Could you check a few things on this model? Use its own coordinates, in mm. A direction names the side the tool comes from. Give positions to 0.01 mm unless a question says otherwise; leave off trailing zeros. Loops run counter-clockwise (first coordinate to the right, second up) from the corner with the lowest first, then second, coordinate; pieces in that order, holes last. Notation, with made-up numbers: (69.5, 2.5) -> (92.5, 2.5) arc R28 cw to (92.5, 24.5) -> close; hole circle Ø2 at (-25.5, -22.75). An arc over 180 degrees is marked (long way). Write item = value, one per line. Start each with the question number.
1) I need wall thicknesses on probe 1 along Z at (x, y) = (19.5, -1.3) (3 decimals); probe 2 along X at (y, z) = (-1, -124) (3 decimals); probe 3 along X at (y, z) = (-2.6, -128) (3 decimals). Which ranges of each line are inside material? Lowest first, please. Write a range as from..to.
2) I want a section at B-B (x = -106). List the corners of the cut face in (y, z) for me (3 decimals).
3) On a 3-axis mill with a long thin cutter (end or side, diameter ignored), from which of +Z, -Z, +X, -X, +Y, -Y can I reach the whole of each face in a straight line? I mean faces 1 (the face through (77.401, -1.565, -75.264)), 2 (the face through (265.049, -1.565, -262.944)). Say none if no direction works.
4) I'm going to push flat-ended pins straight in: pin 1 Ø1.6 at (x, y) = (-361, -1) entering from +Z (3 decimals); pin 2 Ø6 at (x, z) = (-29, -121.5) entering from -Y (3 decimals). Where does each tip first touch, or does it pass through?
5) If we mould it in two halves opening along Z, with no side actions, what happens to faces 3 (the face through (-75.264, -1.565, -77.401)), 4 (the face through (262.944, -1.565, 265.049)), 5 (the face through (79, -3.175, -89))? For each: +Z half, -Z half, draft (parallel to the pull), parting line (faces both ways), or undercut.
6) I want a section at C-C (z = 65). List the corners of the cut face in (x, y) for me (3 decimals), and give its area (3 significant figures).
7) I want a section at D-D (x = -221.5). List the corners of the cut face in (y, z) for me (3 decimals), and give its area (3 significant figures).
8) I want a section at A-A (y = -2.3). List the corners of the cut face in (x, z) for me (3 decimals).
from build123d import *

# Parameters (mm, degrees)
SKETCH2_W           = 755.65
SKETCH2_H           = 755.65
BASE_FLANGE1_DEPTH  = 3.175
CUT_EXTRUDE1_DEPTH  = 535.334672162
CUT_EXTRUDE2_DEPTH  = 535.334672162
BREAK_CORNER1_START = -3.175
BREAK_CORNER1_DEPTH = 3.175


# Read off the part's stored shape, not the designer's step: Break-Corner1
# Sheet-metal steps are written as plain solids
with BuildPart() as part:
    # Sketch2 → Base-Flange1 (new body)
    with BuildSketch(Plane(origin=(0, 0, 0), x_dir=(1, 0, 0), z_dir=(0, 1, 0))):
        Rectangle(SKETCH2_W, SKETCH2_H)
    extrude(amount=-BASE_FLANGE1_DEPTH)

    # Sketch3 → Cut-Extrude1 (cut, through all)
    with BuildSketch(Plane(origin=(0, 0, 0), x_dir=(1, 0, 0), z_dir=(0, 1, 0))):
        Polygon((0, -152.664354058), (152.664354058, 0), (0, 152.664354058), (-152.664354058, 0), align=None)
    extrude(amount=-CUT_EXTRUDE1_DEPTH, mode=Mode.SUBTRACT)

    # Sketch4 → Cut-Extrude2 (cut, through all)
    with BuildSketch(Plane(origin=(0, 0, 0), x_dir=(1, 0, 0), z_dir=(0, 1, 0))):
        with BuildLine():
            Line((377.825, 206.375), (352.425, 206.375))
            ThreePointArc((352.425, 206.375), (263.993664919, 263.993664919), (206.375, 352.425))
            Line((206.375, 352.425), (206.375, 377.825))
            Line((206.375, 377.825), (377.825, 377.825))
            Line((377.825, 377.825), (377.825, 206.375))
        make_face()
        with BuildLine():
            Line((206.375, -377.825), (206.375, -352.425))
            ThreePointArc((206.375, -352.425), (263.993664919, -263.993664919), (352.425, -206.375))
            Line((352.425, -206.375), (377.825, -206.375))
            Line((377.825, -206.375), (377.825, -377.825))
            Line((377.825, -377.825), (206.375, -377.825))
        make_face()
        with BuildLine():
            Line((-377.825, -206.375), (-352.425, -206.375))
            ThreePointArc((-352.425, -206.375), (-263.993664919, -263.993664919), (-206.375, -352.425))
            Line((-206.375, -352.425), (-206.375, -377.825))
            Line((-206.375, -377.825), (-377.825, -377.825))
            Line((-377.825, -377.825), (-377.825, -206.375))
        make_face()
        with BuildLine():
            Line((-206.375, 377.825), (-206.375, 352.425))
            ThreePointArc((-206.375, 352.425), (-263.993664919, 263.993664919), (-352.425, 206.375))
            Line((-352.425, 206.375), (-377.825, 206.375))
            Line((-377.825, 206.375), (-377.825, 377.825))
            Line((-377.825, 377.825), (-206.375, 377.825))
        make_face()
    extrude(amount=-CUT_EXTRUDE2_DEPTH, mode=Mode.SUBTRACT)

    # Break-Corner1 outline → Break-Corner1 (cut)
    with BuildSketch(Plane(origin=(0, 0, 0), x_dir=(1, 0, 0), z_dir=(0, 1, 0)).offset(BREAK_CORNER1_START)):
        Polygon((-206.375, 374.65), (-203.2, 377.825), (-206.375, 377.825), align=None)
        Polygon((203.2, 377.825), (206.375, 374.65), (206.375, 377.825), align=None)
        Polygon((377.825, -206.375), (377.825, -203.2), (374.65, -206.375), align=None)
        Polygon((374.65, 206.375), (377.825, 203.2), (377.825, 206.375), align=None)
        Polygon((-374.65, -206.375), (-377.825, -203.2), (-377.825, -206.375), align=None)
        Polygon((-377.825, 203.2), (-374.65, 206.375), (-377.825, 206.375), align=None)
        Polygon((206.375, -374.65), (203.2, -377.825), (206.375, -377.825), align=None)
        Polygon((-203.2, -377.825), (-206.375, -374.65), (-206.375, -377.825), align=None)
    extrude(amount=BREAK_CORNER1_DEPTH, mode=Mode.SUBTRACT)


solid = part.part
Answer list:
q1.probe_1 = -377.825..-133.164, 133.164..377.825
q1.probe_2 = -377.825..-28.664, 28.664..377.825
q1.probe_3 = -377.825..-24.664, 24.664..377.825
q2.outline = (-3.175, -377.825) -> (0, -377.825) -> (0, -46.664) -> (-3.175, -46.664) -> close; (-3.175, 46.664) -> (0, 46.664) -> (0, 377.825) -> (-3.175, 377.825) -> close
q3.face_1 = +Y, -Y
q3.face_2 = -Z, +X, +Y, -Y
q4.pin_1 = 206.375
q4.pin_2 = -3.175
q5.face_3 = undercut
q5.face_4 = +Z half
q5.face_5 = draft
q6.outline = (-377.825, -3.175) -> (-87.664, -3.175) -> (-87.664, 0) -> (-377.825, 0) -> close; (87.664, -3.175) -> (377.825, -3.175) -> (377.825, 0) -> (87.664, 0) -> close
q6.area = 1,840 mm^2
q7.outline = (-3.175, -320.229) -> (0, -320.229) -> (0, 320.229) -> (-3.175, 320.229) -> close
q7.area = 2,030 mm^2
q8.outline = (-377.825, -203.2) -> (-374.65, -206.375) -> (-352.425, -206.375) arc R255.647 cw to (-206.375, -352.425) -> (-206.375, -374.65) -> (-203.2, -377.825) -> (203.2, -377.825) -> (206.375, -374.65) -> (206.375, -352.425) arc R255.647 cw to (352.425, -206.375) -> (374.65, -206.375) -> (377.825, -203.2) -> (377.825, 203.2) -> (374.65, 206.375) -> (352.425, 206.375) arc R255.647 cw to (206.375, 352.425) -> (206.375, 374.65) -> (203.2, 377.825) -> (-203.2, 377.825) -> (-206.375, 374.65) -> (-206.375, 352.425) arc R255.647 cw to (-352.425, 206.375) -> (-374.65, 206.375) -> (-377.825, 203.2) -> close; hole (-152.664, 0) -> (0, -152.664) -> (152.664, 0) -> (0, 152.664) -> close
